from build123d import *

# Parameters (mm, degrees)
F0_W      = 70
F0_H      = 135
F1_DEPTH  = 10
F2_T      = -2.5
F3_R      = 5
F4_R      = 5
F5_R      = 5
F6_R      = 5
F7_W      = 1
F7_H      = 4
F8_DEPTH  = 1
F9_W      = 30
F9_H      = 2
F9_W_2    = 15
F10_DEPTH = 4
F12_W     = 30
F12_H     = 14
F12_H_2   = 2
F13_DEPTH = 1
F11_W     = 30
F11_H     = 2
F11_H_2   = 14
F14_DEPTH = 1


with BuildPart() as f1:
    # F0 (on Top) → F1 (new body)
    with BuildSketch(Plane.XY):
        Rectangle(F0_W, F0_H)
    extrude(amount=F1_DEPTH)

    # F2
    f2_openings = [f1.faces().sort_by_distance(p)[0] for p in [
        (0, 0, 0),
    ]]
    offset(amount=F2_T, openings=f2_openings)

    # F3
    f3_edges = [f1.edges().sort_by_distance(p)[0] for p in [
        (0, 67.5, 10),
        (35, 0, 10),
        (35, 67.5, 5),
    ]]
    fillet(f3_edges, radius=F3_R)

    # F4
    f4_edges = [f1.edges().sort_by_distance(p)[0] for p in [
        (33.535534, -67.5, 8.535534),
        (-2.5, -67.5, 10),
    ]]
    fillet(f4_edges, radius=F4_R)

    # F5
    f5_edges = [f1.edges().sort_by_distance(p)[0] for p in [
        (-35, 0, 10),
        (-35, -66.035534, 8.535534),
    ]]
    fillet(f5_edges, radius=F5_R)

    # F6
    f6_edges = [f1.edges().sort_by_distance(p)[0] for p in [
        (32.5, 65, 3.75),
        (-32.5, 65, 3.75),
        (32.5, -65, 3.75),
        (-32.5, -65, 3.75),
    ]]
    fillet(f6_edges, radius=F6_R)

    # F7 (on face) → F8 (cut)
    with BuildSketch(Plane(origin=(0, 0, 0), x_dir=(1, 0, 0), z_dir=(0, 0, -1))):
        with Locations((-33.75, 0)):
            Rectangle(F7_W, F7_H)
        with Locations((33.75, 0)):
            Rectangle(F7_W, F7_H)
    extrude(amount=-F8_DEPTH, mode=Mode.SUBTRACT)

    # F9 (on face) → F10 (join)
    with BuildSketch(Plane.XY.offset(10)):
        with Locations((0, 38.25)):
            Rectangle(F9_W, F9_H)
        with Locations((-7.5, -38.25)):
            Rectangle(F9_W_2, F9_H)
        with Locations((7.5, -38.25)):
            Rectangle(F9_W_2, F9_H)
    extrude(amount=F10_DEPTH)

    # F12 (on face) → F13 (join)
    with BuildSketch(Plane.XY.offset(14)):
        with Locations((0, -30.25)):
            Rectangle(F12_W, F12_H)
        with Locations((0, -38.25)):
            Rectangle(F12_W, F12_H_2)
    extrude(amount=F13_DEPTH)

    # F11 (on face) → F14 (join)
    with BuildSketch(Plane.XY.offset(14)):
        with Locations((0, 38.25)):
            Rectangle(F11_W, F11_H)
        with Locations((0, 30.25)):
            Rectangle(F11_W, F11_H_2)
    extrude(amount=F14_DEPTH)


solid = f1.part
Model file for the job. Use its own axes, mm. A direction names the side the tool comes from. Coordinates: 2 decimals unless noted, no trailing zeros. Order: outer loops, then holes, each group sorted by start corner. A loop starts at its lowest first (then second) coordinate and runs counter-clockwise, first axis right, second up. Notation, with made-up numbers: (37, -20.5) -> (64, -20.5) arc R29 cw to (64, 16.5) -> close; hole circle Ø4 at (43, 81). An arc over 180 degrees is marked (long way). Return JSON: item names as keys, results as strings. Group by question number.
Item 1: Saw through at A-A on y = 27. Write the cut outline in (x, z), then the cut area to 3 significant figures.
Item 2: Saw through at D-D on y = -56.5. Write the cut outline in (x, z).
Item 3: Flat gauge pins, fed straight in: P1, Ø8, axis at y = 17.5, z = 12.5, coming from the -X side; P2, Ø1.5, axis at x = 25, z = 11, coming from the +Y side; P3, Ø5, axis at x = 2.5, y = 5.5, coming from the -Z side; P4, Ø8, axis at x = -18, z = 13, coming from the +Y side. Where does each tip first touch, or does it go through?
Item 4: Saw through at C-C on x = -25.5. Write the cut outline in (y, z).
Item 5: Tool access for faces 4 (the flat face through (32.5, -1, 4)), 5 (the flat face through (0, -39.25, 12)), 6 (the flat face through (0, 39.25, 12)): list every direction of +Z, -Z, +X, -X, +Y, -Y with a clear straight run to the whole face (end or side of a thin tool).
Item 6: Pull direction Z, two halves, no side cores. Call faces 1 (the cylindrical face through (-34, 1, 8)), 2 (the flat face through (0, -67.5, 2)), 3 (the flat face through (0, -37.25, 12)): pulls with the +Z half, pulls with the -Z half, needs draft (parallel to the pull), parting line crosses it, or undercut.
Item 7: Wall check: line 1 along Z through (x, y) = (-13, 30); line 2 along X through (y, z) = (-24.5, 2.25); line 3 along Y through (x, z) = (-14, 10.75). Give the ranges that are in metal, low to high. Write a range as [from, to].
Item 8: Saw through at B-B on z = 11.5. Write the cut outline in (x, y).
Values found:
{
 "1": {"outline": "(-35, 0) -> (-32.5, 0) -> (-32.5, 7.5) -> (32.5, 7.5) -> (32.5, 0) -> (35, 0) -> (35, 5) arc R5 ccw to (30, 10) -> (-30, 10) arc R5 ccw to (-35, 5) -> close; (-15, 14) -> (15, 14) -> (15, 15) -> (-15, 15) -> close", "area": "232 mm2"},
 "2": {"outline": "(-35, 0) -> (-32.5, 0) -> (-32.5, 7.5) -> (32.5, 7.5) -> (32.5, 0) -> (35, 0) -> (35, 5) arc R5 ccw to (30, 10) -> (-30, 10) arc R5 ccw to (-35, 5) -> close"},
 "3": {"P1": "stops at x = -33.57", "P2": "passes through", "P3": "stops at z = 7.5", "P4": "stops at y = 65.5"},
 "4": {"outline": "(-67.5, 0) -> (-65, 0) -> (-65, 7.5) -> (65, 7.5) -> (65, 0) -> (67.5, 0) -> (67.5, 5) arc R5 ccw to (62.5, 10) -> (-62.5, 10) arc R5 ccw to (-67.5, 5) -> close"},
 "5": {"face 4": "-Z", "face 5": "+Z, +X, -X, -Y", "face 6": "+Z, +X, -X, +Y"},
 "6": {"face 1": "pulls with the +Z half", "face 2": "needs draft", "face 3": "undercut"},
 "7": {"line 1": "z = [7.5, 10], [14, 15]", "line 2": "x = [-35, -32.5], [32.5, 35]", "line 3": "y = [-39.25, -37.25], [37.25, 39.25]"},
 "8": {"outline": "(-15, -39.25) -> (15, -39.25) -> (15, -37.25) -> (-15, -37.25) -> close; (-15, 37.25) -> (15, 37.25) -> (15, 39.25) -> (-15, 39.25) -> close"}
}
